Geometry: final body of the model. Coordinates: model frame, mm. Round coordinates to 2 decimals unless told otherwise and drop trailing zeros. Loops run counter-clockwise (first coordinate to the right, second up) from the corner with the lowest first, then second, coordinate; pieces in that order, holes last. Notation, with made-up numbers: (53.5, 2.25) - (76.5, 2.25) arc R7 cw to (76.5, 11.25) - close; hole circle Ø8 at (-33, 38). An arc over 180 degrees is marked (long way). Answer as a JSON object with one key per item and string values. Group by question number.
Item 1: Section B-B (y = 0). Return the cut outline in (x, z) (3 decimals).
Item 2: Section A-A (x = 0). Return the cut outline in (y, z) (3 decimals).
Item 3: First-contact query: pin 1 (1 mm diameter, centred on x = 195.5, z = 2, fed in from +Y); pin 2 (1 mm diameter, centred on x = 47, z = 2.5, fed in from -Y). Flat tips, straight axial feed; report the tip coordinate or a pass-through.
Item 4: Section C-C (z = 1.75). Return the cut outline in (x, y) (3 decimals), plus the area to 3 significant figures.
Item 5: Line query: line 1 (Y direction, x = 0, z = 1.85) (3 decimals); line 2 (X direction, y = 3, z = 0.45); line 3 (Y direction, x = 49.5, z = 2.45) (3 decimals). Output: solid intervals per line, ascending.
Item 6: Section D-D (x = 190.5). Return the cut outline in (y, z) (3 decimals).
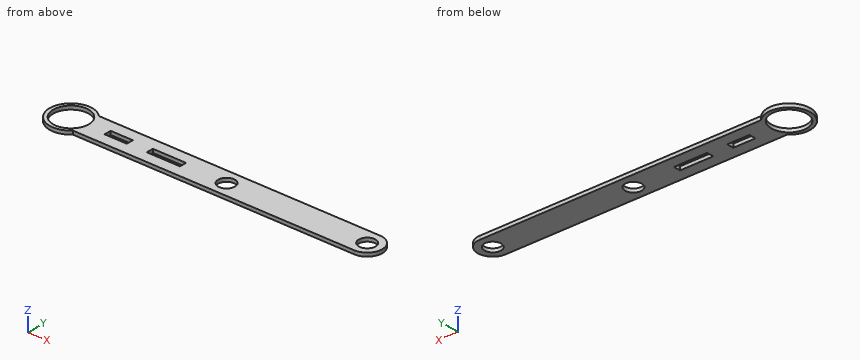
```python
from build123d import *

# Parameters (mm, degrees)
SKETCH1_R           = 15.875
SKETCH1_R_2         = 7.5
SKETCH1_W           = 20
SKETCH1_H           = 6.35
SKETCH1_W_2         = 30
BOSS_EXTRUDE1_DEPTH = 3.175


with BuildPart() as part:
    # Sketch1 → Boss-Extrude1 (new body)
    with BuildSketch(Plane.XY):
        with BuildLine():
            Line((13.470384182, 13.470384182), (267.470384182, 13.470384182))
            ThreePointArc((267.470384182, 13.470384182), (280.940768363, 0), (267.470384182, -13.470384182))
            Line((267.470384182, -13.470384182), (13.470384182, -13.470384182))
            ThreePointArc((13.470384182, -13.470384182), (-19.05, 0), (13.470384182, 13.470384182))
        make_face()
        Circle(SKETCH1_R, mode=Mode.SUBTRACT)
        with Locations((267.470384182, 0)):
            Circle(SKETCH1_R_2, mode=Mode.SUBTRACT)
        with Locations((140.470384182, 0)):
            Circle(SKETCH1_R_2, mode=Mode.SUBTRACT)
        with Locations((43.11714777, 0)):
            Rectangle(SKETCH1_W, SKETCH1_H, mode=Mode.SUBTRACT)
        with Locations((86.195594821, 0)):
            Rectangle(SKETCH1_W_2, SKETCH1_H, mode=Mode.SUBTRACT)
    extrude(amount=BOSS_EXTRUDE1_DEPTH)


solid = part.part
```
Values:
{
 "1": {"outline": "(-19.05, 0) - (-15.875, 0) - (-15.875, 3.175) - (-19.05, 3.175) - close; (15.875, 0) - (33.117, 0) - (33.117, 3.175) - (15.875, 3.175) - close; (53.117, 0) - (71.196, 0) - (71.196, 3.175) - (53.117, 3.175) - close; (101.196, 0) - (132.97, 0) - (132.97, 3.175) - (101.196, 3.175) - close; (147.97, 0) - (259.97, 0) - (259.97, 3.175) - (147.97, 3.175) - close; (274.97, 0) - (280.941, 0) - (280.941, 3.175) - (274.97, 3.175) - close"},
 "2": {"outline": "(-19.05, 0) - (-15.875, 0) - (-15.875, 3.175) - (-19.05, 3.175) - close; (15.875, 0) - (19.05, 0) - (19.05, 3.175) - (15.875, 3.175) - close"},
 "3": {"pin 1": "stops at y = 13.47", "pin 2": "stops at y = -13.47"},
 "4": {"outline": "(13.47, -13.47) - (267.47, -13.47) arc R13.47 ccw to (267.47, 13.47) - (13.47, 13.47) arc R19.05 ccw (long way) to start; hole circle Ø31.75 at (0, 0); hole (33.117, -3.175) - (53.117, -3.175) - (53.117, 3.175) - (33.117, 3.175) - close; hole (71.196, -3.175) - (101.196, -3.175) - (101.196, 3.175) - (71.196, 3.175) - close; hole circle Ø15 at (140.47, 0); hole circle Ø15 at (267.47, 0)", "area": "6,700 mm^2"},
 "5": {"line 1": "y = -19.05 to -15.875, 15.875 to 19.05", "line 2": "x = -18.81 to -15.59, 15.59 to 33.12, 53.12 to 71.2, 101.2 to 133.6, 147.34 to 260.6, 274.34 to 280.6", "line 3": "y = -13.47 to -3.175, 3.175 to 13.47"},
 "6": {"outline": "(-13.47, 0) - (13.47, 0) - (13.47, 3.175) - (-13.47, 3.175) - close"}
}
